from build123d import *

# Parameters (mm, degrees)
F1_DEPTH = 1.5
F2_R     = 17.5
F3_DEPTH = 1.501
F4_W     = 2.75
F4_H     = 1.5
F5_DEPTH = 8
F7_DEPTH = 1.501


with BuildPart() as f1:
    # F0 (on Front) → F1 (new body)
    with BuildSketch(Plane.XZ):
        with BuildLine():
            ThreePointArc((-25.8904117895, 42.4818245173), (-38.971887268, 10.9003490722), (-7.3904118091, 23.9818245173))
            ThreePointArc((-7.3904118091, 23.9818245173), (-12.8089363502, 37.0632999623), (-25.8904117895, 42.4818245173))
        make_face()
        with BuildLine():
            ThreePointArc((11.1095881909, 42.4818245173), (-1.971887261, 37.0632999692), (-7.3904118091, 23.9818245173))
            ThreePointArc((-7.3904118091, 23.9818245173), (11.1095881909, 5.4818245173), (29.6095881909, 23.9818245173))
            ThreePointArc((29.6095881909, 23.9818245173), (24.1910636429, 37.0632999692), (11.1095881909, 42.4818245173))
        make_face()
        with BuildLine():
            ThreePointArc((-25.8904117895, 42.4818245173), (-12.8089363502, 37.0632999623), (-7.3904118091, 23.9818245173))
            ThreePointArc((-7.3904118091, 23.9818245173), (-1.971887261, 37.0632999692), (11.1095881909, 42.4818245173))
            ThreePointArc((11.1095881909, 42.4818245173), (-1.971887261, 47.9003490653), (-7.3904118091, 60.9818245173))
            ThreePointArc((-7.3904118091, 60.9818245173), (-12.8089363502, 47.9003490722), (-25.8904117895, 42.4818245173))
        make_face()
        with BuildLine():
            ThreePointArc((-7.3904118091, 60.9818245173), (-38.971887268, 74.0632999623), (-25.8904117895, 42.4818245173))
            ThreePointArc((-25.8904117895, 42.4818245173), (-12.8089363502, 47.9003490722), (-7.3904118091, 60.9818245173))
        make_face()
        with BuildLine():
            ThreePointArc((-7.3904118091, 60.9818245173), (-1.971887261, 47.9003490653), (11.1095881909, 42.4818245173))
            ThreePointArc((11.1095881909, 42.4818245173), (24.1910636429, 47.9003490653), (29.6095881909, 60.9818245173))
            ThreePointArc((29.6095881909, 60.9818245173), (11.1095881909, 79.4818245173), (-7.3904118091, 60.9818245173))
        make_face()
    extrude(amount=F1_DEPTH)

    # F2 (on face) → F3 (cut, through all)
    with BuildSketch(Plane.XZ.offset(1.5)):
        with Locations((-25.8904118091, 60.9818245173)):
            Circle(F2_R)
        with Locations((-25.8904118091, 23.9818245173)):
            Circle(F2_R)
        with Locations((11.1095881909, 60.9818245173)):
            Circle(F2_R)
        with Locations((11.1095881909, 23.9818245173)):
            Circle(F2_R)
    extrude(amount=-F3_DEPTH, mode=Mode.SUBTRACT)

    # F4 (on face) → F5 (join)
    with BuildSketch(Plane.XZ.offset(1.5)):
        with Locations((-6.0154118091, 34.3318245173)):
            Rectangle(F4_W, F4_H)
        with Locations((-8.7654118091, 34.3318245173)):
            Rectangle(F4_W, F4_H)
        with Locations((-8.7654118091, 50.6318245173)):
            Rectangle(F4_W, F4_H)
        with Locations((-6.0154118091, 50.6318245173)):
            Rectangle(F4_W, F4_H)
    extrude(amount=F5_DEPTH)

    # F6 (on face) → F7 (cut, through all)
    with BuildSketch(Plane.XZ.offset(1.5)):
        with BuildLine():
            ThreePointArc((-12.7348604006, 45.4258701055), (-16.5319645782, 42.4818245173), (-12.7348604006, 39.537778929))
            ThreePointArc((-12.7348604006, 39.537778929), (-7.3893052189, 36.3801416389), (-2.0448957156, 39.5397176417))
            ThreePointArc((-2.0448957156, 39.5397176417), (1.7489974946, 42.4818245173), (-2.0448957156, 45.4239313928))
            ThreePointArc((-2.0448957156, 45.4239313928), (-7.3893052189, 48.5835073956), (-12.7348604006, 45.4258701055))
        make_face()
    extrude(amount=-F7_DEPTH, mode=Mode.SUBTRACT)


solid = f1.part
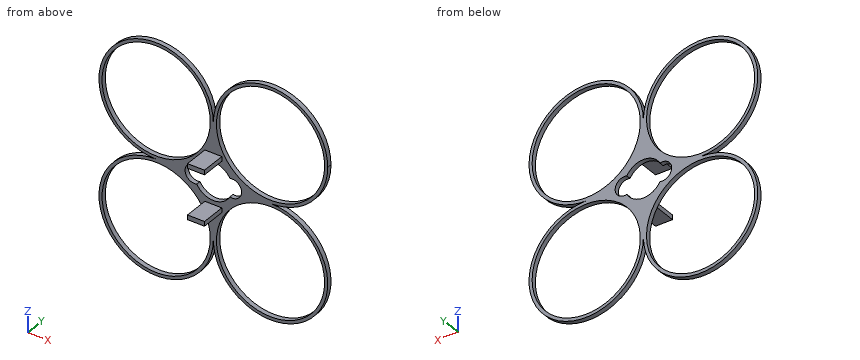
Work out the finished part from the listing and answer in its coordinate system (mm). Round coordinates to 2 decimals unless told otherwise and drop trailing zeros. Write each loop counter-clockwise with the first axis right and the second up, starting at its lowest first coordinate (ties: lowest second). Pieces come first, ordered by that corner, then holes.
1) Given pin 1 Ø1.2 at (y, z) = (-6, 34.5) entering from -X; pin 2 Ø1.6 at (y, z) = (-4, 50.5) entering from +X; pin 3 Ø3 at (x, y) = (-6, -5) entering from +Z; pin 4 Ø21 at (x, z) = (11.11, 60.98) entering from -Y, each flat-ended and moving along its own axis, determine where each tip first touches the part or whether it passes through.
2) Straight lines are drawn through the part: line 1 (Z direction, x = -35, y = -1.25); line 2 (X direction, y = -0.5, z = 38.5); line 3 (X direction, y = -0.5, z = 17). For each, find the intervals that lie inside material, in ascending order.
3) A cutting plane is placed at A-A (y = -6). Give the vertices of the cut face in (x, z).
4) A cutting plane is placed at B-B (x = 23.5). Give the vertices of the cut face in (y, z), plus the area to 3 significant figures.
5) A cutting plane is placed at D-D (x = -24). Give the vertices of the cut face in (y, z).
6) A cutting plane is placed at C-C (z = 64.5). Give the vertices of the cut face in (x, y).
Completed:
1. pin 1: stops at x = -10.14
1. pin 2: stops at x = -4.64
1. pin 3: stops at z = 51.38
1. pin 4: passes through
2. line 1: z = 7.88 to 9.04, 38.92 to 40.08, 44.88 to 46.04, 75.92 to 77.08
2. line 2: x = -37.36 to -35.66, -16.12 to -12.01, -2.77 to 1.34, 20.88 to 22.58
2. line 3: x = -43.02 to -41.94, -9.84 to -8.76, -6.02 to -4.94, 27.16 to 28.24
3. outline: (-10.14, 33.58) - (-4.64, 33.58) - (-4.64, 35.08) - (-10.14, 35.08) - close; (-10.14, 49.88) - (-4.64, 49.88) - (-4.64, 51.38) - (-10.14, 51.38) - close
4. outline: (-1.5, 10.24) - (0, 10.24) - (0, 11.62) - (-1.5, 11.62) - close; (-1.5, 36.34) - (0, 36.34) - (0, 37.72) - (-1.5, 37.72) - close; (-1.5, 47.24) - (0, 47.24) - (0, 48.62) - (-1.5, 48.62) - close; (-1.5, 73.34) - (0, 73.34) - (0, 74.72) - (-1.5, 74.72) - close
4. area: 8.28 mm2
5. outline: (-1.5, 5.58) - (0, 5.58) - (0, 6.58) - (-1.5, 6.58) - close; (-1.5, 41.38) - (0, 41.38) - (0, 43.58) - (-1.5, 43.58) - close; (-1.5, 78.38) - (0, 78.38) - (0, 79.38) - (-1.5, 79.38) - close
6. outline: (-44.05, -1.5) - (-43.03, -1.5) - (-43.03, 0) - (-44.05, 0) - close; (-8.75, -1.5) - (-7.73, -1.5) - (-7.73, 0) - (-8.75, 0) - close; (-7.05, -1.5) - (-6.03, -1.5) - (-6.03, 0) - (-7.05, 0) - close; (28.25, -1.5) - (29.27, -1.5) - (29.27, 0) - (28.25, 0) - close
